Source: CAD feature listing. Evaluate the final solid. Frame: model axes, mm. Face numbers are marked on the shaded views. A direction names the side the tool comes from. Coordinates: 2 decimals unless noted, no trailing zeros. Order: outer loops, then holes, each group sorted by start corner. A loop starts at its lowest first (then second) coordinate and runs counter-clockwise, first axis right, second up. Notation, with made-up numbers: (83.5, 25) -> (119.5, 25) arc R12 ccw to (119.5, 41) -> close; hole circle Ø3 at (17, 78). An arc over 180 degrees is marked (long way). Write each question's results on one line, items separated by ' | '. Start each with the question number.
from build123d import *

# Parameters (mm, degrees)
F0_R     = 29.05
F0_R_2   = 19.05
F1_DEPTH = 50.8
F2_W     = 26.768681
F2_H     = 10.474702
F3_DEPTH = 50.8


with BuildPart() as f1:
    # F0 (on Top) → F1 (new body)
    with BuildSketch(Plane.XY):
        Circle(F0_R)
        Circle(F0_R_2, mode=Mode.SUBTRACT)
    extrude(amount=F1_DEPTH)


with BuildPart() as f3:
    # F2 (on Front) → F3 (new body, symmetric)
    with BuildSketch(Plane.XZ):
        with Locations((1.88487, 32.046725)):
            Rectangle(F2_W, F2_H)
    extrude(amount=F3_DEPTH, both=True)


with BuildPart() as f1_1:
    add(f1.part)

    # F4: cut F3
    add(f3.part, mode=Mode.SUBTRACT)


solid = f1_1.part
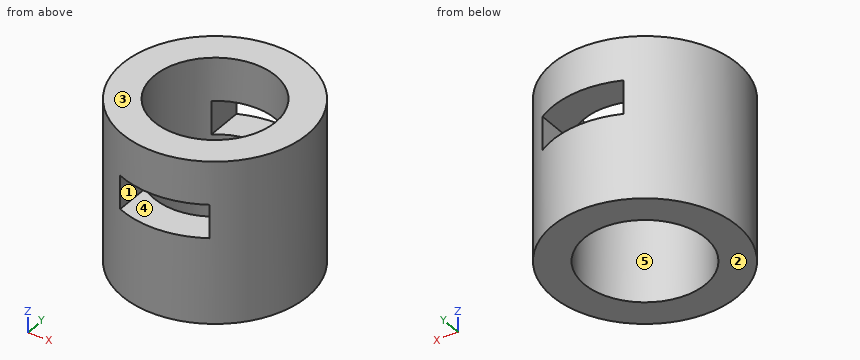
(1) Draft query along Z for the marked faces 1, 2 and 3. Return one class per face: released by +Z, released by -Z, zero draft, split by the parting line, or undercut.
(2) Section B-B on y = 0. Return the cut outline in (x, z), then the cut area to 3 significant figures.
(3) Section D-D on z = 15.5. Return the cut outline in (x, y).
(4) Reachability of the marked faces 4 and 5 from +Z, -Z, +X, -X, +Y, -Y: full face, straight path, thin tool, end or side. Return the list, or none.
(5) Section A-A on x = 0. Return the cut outline in (y, z).
(6) Section C-C on y = -17.5. Return the cut outline in (x, z).
(7) Line query: L1, parallel to Z at x = 1, y = -22; L2, parallel to Y at x = 0, z = 14; L3, parallel to X at y = 3, z = 17.5. Output: solid intervals per line, ascending.
(8) First-contact query: P1, Ø9, axis at x = -2, y = -17, coming from the +Z side; P2, Ø3, axis at y = -15, z = 31.5, coming from the -X side; P3, Ø8, axis at y = -8.5, z = 42.5, coming from the -X side; P4, Ø5, axis at y = 18, z = 32.5, coming from the -X side. Flat tips, straight axial feed; report the tip coordinate or a pass-through.
Results list:
1) face 1: undercut | face 2: released by -Z | face 3: released by +Z
2) outline: (-29.05, 0) -> (-19.05, 0) -> (-19.05, 50.8) -> (-29.05, 50.8) -> close; (19.05, 0) -> (29.05, 0) -> (29.05, 50.8) -> (19.05, 50.8) -> close | area: 1,020 mm²
3) outline: circle Ø58.1 at (0, 0); hole circle Ø38.1 at (0, 0)
4) face 4: +Y, -Y | face 5: +Z, -Z
5) outline: (-29.05, 0) -> (-19.05, 0) -> (-19.05, 26.81) -> (-29.05, 26.81) -> close; (-29.05, 37.28) -> (-19.05, 37.28) -> (-19.05, 50.8) -> (-29.05, 50.8) -> close; (19.05, 0) -> (29.05, 0) -> (29.05, 26.81) -> (19.05, 26.81) -> close; (19.05, 37.28) -> (29.05, 37.28) -> (29.05, 50.8) -> (19.05, 50.8) -> close
6) outline: (-23.19, 0) -> (-7.53, 0) -> (-7.53, 26.81) -> (-11.5, 26.81) -> (-11.5, 37.28) -> (-7.53, 37.28) -> (-7.53, 50.8) -> (-23.19, 50.8) -> close; (7.53, 0) -> (23.19, 0) -> (23.19, 50.8) -> (7.53, 50.8) -> (7.53, 37.28) -> (15.27, 37.28) -> (15.27, 26.81) -> (7.53, 26.81) -> close
7) L1: z = 0 to 26.81, 37.28 to 50.8 | L2: y = -29.05 to -19.05, 19.05 to 29.05 | L3: x = -28.89 to -18.81, 18.81 to 28.89
8) P1: stops at z = 50.8 | P2: stops at x = -25.72 | P3: stops at x = -28.7 | P4: stops at x = -24.57
